For this review, use the dimensioned drawing (mm, ordinates from the lowest corner) and the shaded views. A direction names the side the tool comes from. Give positions to 0.01 mm unless a question says otherwise; leave off trailing zeros. Order: outer loops, then holes, each group sorted by start corner. A loop starts at its lowest first (then second) coordinate and runs counter-clockwise, first axis right, second up. Notation, with made-up numbers: (-35, 16.25) -> (7, 16.25) arc R8 cw to (7, 31.25) -> close; hole circle Ø3 at (-31, 39.5). An arc over 180 degrees is marked (long way). One line per item, written item: value. Start each with the question number.
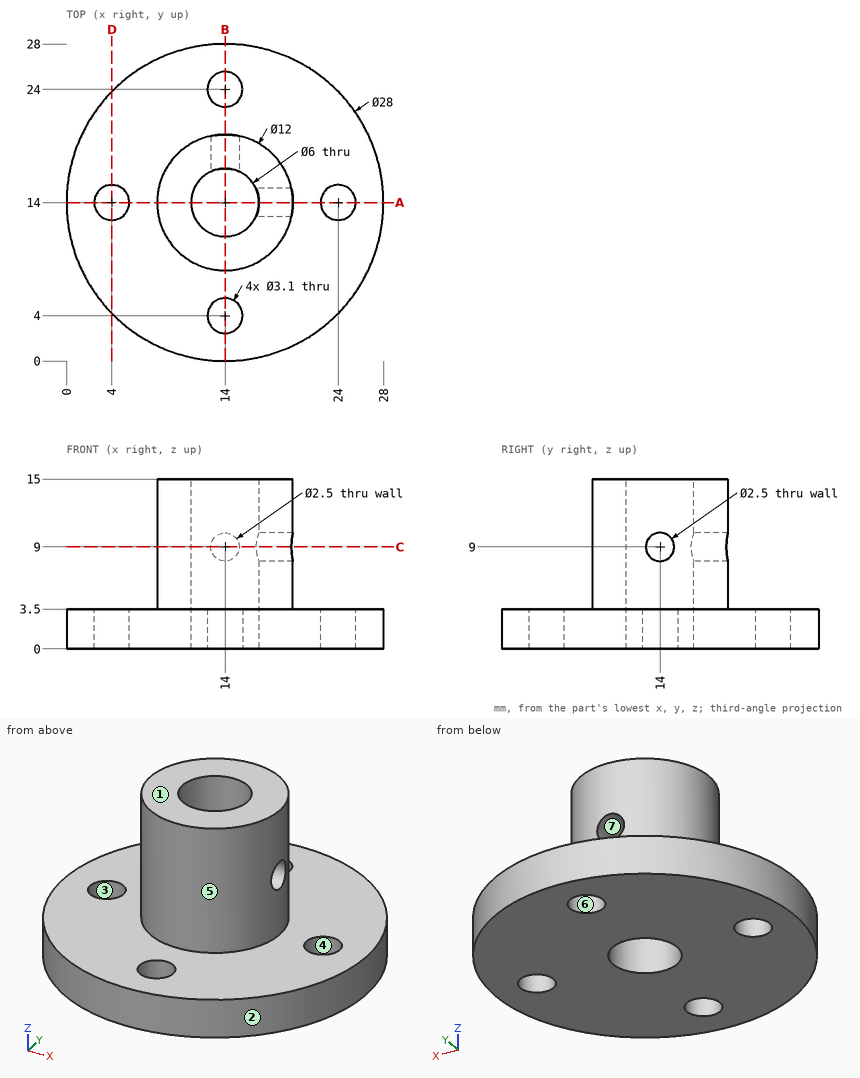
Q1. Take a section at C-C (z = 9). State the section outline as (x, y) points, and give its area (3 significant figures).
Q2. Take a section at A-A (y = 14). State the section outline as (x, z) points.
Q3. Take a section at D-D (x = 4). State the section outline as (y, z) points.
Q4. Mouldability with a two-part tool opening along X and no side actions: class the marked faces 1, 2, 3 and 4 as pulls with the +X half, pulls with the -X half, needs draft (parallel to the pull), parting line crosses it, or undercut.
Q5. For pin 1 Ø5 at (x, y) = (4, 14) entering from +Z; pin 2 Ø8 at (y, z) = (8, 12.5) entering from -X; pin 3 Ø3 at (y, z) = (14, 9) entering from +X, all flat-tipped, find the tip position at first contact; note any pin that passes through.
Q6. For line 1 along Z through (x, y) = (17.6, 14); line 2 along Y through (x, z) = (14, 4.5); line 3 along Z through (x, y) = (18.25, 3), list the stretches that pass through material, from the lowest coordinate up.
Q7. For the marked faces 5, 6 and 7, list the 3-axis set-ups (+Z, -Z, +X, -X, +Y, -Y) from which the entire face can be reached by the end or side of a thin tool; tool diameter is ignored.
Answers below:
1. outline: (12.75, 16.73) -> (12.75, 19.87) arc R6 ccw (long way) to (19.87, 12.75) -> (16.73, 12.75) arc R3 cw (long way) to start; (15.25, 16.73) arc R3 cw to (16.73, 15.25) -> (19.87, 15.25) arc R6 ccw to (15.25, 19.87) -> close
1. area: 69.6 mm²
2. outline: (0, 0) -> (2.45, 0) -> (2.45, 3.5) -> (0, 3.5) -> close; (5.55, 0) -> (11, 0) -> (11, 15) -> (8, 15) -> (8, 3.5) -> (5.55, 3.5) -> close; (17, 0) -> (22.45, 0) -> (22.45, 3.5) -> (20, 3.5) -> (20, 7.75) -> (17, 7.75) -> close; (17, 10.25) -> (20, 10.25) -> (20, 15) -> (17, 15) -> close; (25.55, 0) -> (28, 0) -> (28, 3.5) -> (25.55, 3.5) -> close
3. outline: (4.2, 0) -> (12.45, 0) -> (12.45, 3.5) -> (4.2, 3.5) -> close; (15.55, 0) -> (23.8, 0) -> (23.8, 3.5) -> (15.55, 3.5) -> close
4. face 1: needs draft
4. face 2: parting line crosses it
4. face 3: undercut
4. face 4: undercut
5. pin 1: stops at z = 3.5
5. pin 2: stops at x = 8.34
5. pin 3: stops at x = 20
6. line 1: z = 0 to 7.75, 10.25 to 15
6. line 2: y = 8 to 11, 17 to 20
6. line 3: z = 0 to 3.5
7. face 5: +Z
7. face 6: +Z, -Z
7. face 7: +Y
